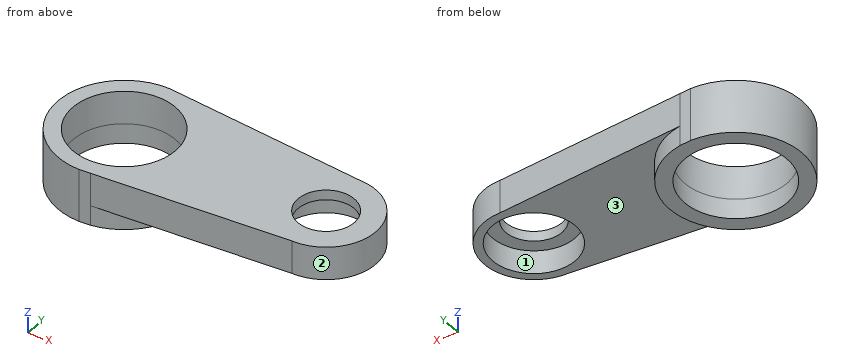
```python
from build123d import *

# Parameters (mm, degrees)
F0_R     = 7.75
F0_R_2   = 6.25
F0_R_3   = 4.25
F1_DEPTH = 5
F2_DEPTH = 3
F3_DEPTH = 3.5


with BuildPart() as f1:
    # F0 (on Top) → F1 (new body)
    with BuildSketch(Plane.XY):
        with BuildLine():
            Line((1.6551724138, 9.8620689655), (0, 10))
            ThreePointArc((0, 10), (-10, 0), (0, -10))
            Line((0, -10), (1.6551724138, -9.8620689655))
            ThreePointArc((1.6551724138, -9.8620689655), (7.6338628537, -6.4594224147), (10, 0))
            ThreePointArc((10, 0), (7.6338628537, 6.4594224147), (1.6551724138, 9.8620689655))
        make_face()
        Circle(F0_R, mode=Mode.SUBTRACT)
        with BuildLine():
            Line((30, 7.5), (1.6551724138, 9.8620689655))
            ThreePointArc((1.6551724138, 9.8620689655), (7.6338628537, 6.4594224147), (10, 0))
            ThreePointArc((10, 0), (7.6338628537, -6.4594224147), (1.6551724138, -9.8620689655))
            Line((1.6551724138, -9.8620689655), (30, -7.5))
            ThreePointArc((30, -7.5), (22.5, 0), (30, 7.5))
        make_face()
        with BuildLine():
            ThreePointArc((37.5, 0), (35.3033008589, 5.3033008589), (30, 7.5))
            ThreePointArc((30, 7.5), (22.5, 0), (30, -7.5))
            ThreePointArc((30, -7.5), (35.3033008589, -5.3033008589), (37.5, 0))
        make_face()
        with Locations((30, 0)):
            Circle(F0_R_2, mode=Mode.SUBTRACT)
        with Locations((30, 0)):
            Circle(F0_R_2)
        with Locations((30, 0)):
            Circle(F0_R_3, mode=Mode.SUBTRACT)
    extrude(amount=F1_DEPTH)

    # F0 (on Top) → F2 (join)
    with BuildSketch(Plane.XY):
        with BuildLine():
            Line((1.6551724138, 9.8620689655), (0, 10))
            ThreePointArc((0, 10), (-10, 0), (0, -10))
            Line((0, -10), (1.6551724138, -9.8620689655))
            ThreePointArc((1.6551724138, -9.8620689655), (7.6338628537, -6.4594224147), (10, 0))
            ThreePointArc((10, 0), (7.6338628537, 6.4594224147), (1.6551724138, 9.8620689655))
        make_face()
        Circle(F0_R, mode=Mode.SUBTRACT)
    extrude(amount=-F2_DEPTH)

    # F0 (on Top) → F3 (cut)
    with BuildSketch(Plane.XY):
        with Locations((30, 0)):
            Circle(F0_R_2)
        with Locations((30, 0)):
            Circle(F0_R_3, mode=Mode.SUBTRACT)
    extrude(amount=F3_DEPTH, mode=Mode.SUBTRACT)


solid = f1.part
```
Read the model definition and answer for the solid it produces. Units are mm, in the model's axes. Face numbers are marked on the shaded views. Give positions to 0.01 mm unless a question says otherwise; leave off trailing zeros. Write each loop counter-clockwise with the first axis right and the second up, starting at its lowest first coordinate (ties: lowest second). Pieces come first, ordered by that corner, then holes. Notation, with made-up numbers: (62, 65.25) -> (115, 65.25) arc R17 ccw to (115, 90.25) -> close; hole circle Ø2 at (73.25, 18). An arc over 180 degrees is marked (long way). Answer in a Markdown table with one row per item.
1) Section D-D on z = -1.5 is taken. Give the vertices of the cut face in (x, y), plus the area to 3 significant figures.
Results list:
| item | result |
|---|---|
| outline | (0, -10) -> (1.66, -9.86) arc R10 ccw to (1.66, 9.86) -> (0, 10) arc R10 ccw to start; hole circle Ø15.5 at (0, 0) |
| area | 125 mm^2 |
2) Section A-A on z = 0.5 is taken. Give the vertices of the cut face in (x, y), plus the area to 3 significant figures.
Results list:
| item | result |
|---|---|
| outline | (0, -10) -> (30, -7.5) arc R7.5 ccw to (30, 7.5) -> (0, 10) arc R10 ccw to start; hole circle Ø15.5 at (0, 0); hole circle Ø12.5 at (30, 0) |
| area | 459 mm^2 |
3) Straight lines are drawn through the part: line 1 (Y direction, x = 30, z = 2.3); line 2 (X direction, y = 5.75, z = 2.5); line 3 (X direction, y = -1.5, z = 0.25). For each, find the intervals that lie inside material, in ascending order. Write a range as [from, to].
Results list:
| item | result |
|---|---|
| line 1 | [-7.5, -6.25], [6.25, 7.5] |
| line 2 | [-8.18, -5.2], [5.2, 27.55], [32.45, 34.82] |
| line 3 | [-9.89, -7.6], [7.6, 23.93], [36.07, 37.35] |
4) Section B-B on y = 2.25 is taken. Give the vertices of the cut face in (x, z).
Results list:
| item | result |
|---|---|
| outline | (-9.74, -3) -> (-7.42, -3) -> (-7.42, 5) -> (-9.74, 5) -> close; (7.42, -3) -> (9.74, -3) -> (9.74, 0) -> (24.17, 0) -> (24.17, 3.5) -> (26.39, 3.5) -> (26.39, 5) -> (7.42, 5) -> close; (33.61, 3.5) -> (35.83, 3.5) -> (35.83, 0) -> (37.15, 0) -> (37.15, 5) -> (33.61, 5) -> close |
5) Each of these flat-tipped pins is pushed along its axis until it touches: pin 1 Ø4 at (x, z) = (-3.5, -0.5) entering from -Y; pin 2 Ø4 at (x, y) = (18, -6.5) entering from -Z; pin 3 Ø1.5 at (y, z) = (5, 0) entering from +X. Where does it stop, or does it pass through?
Results list:
| item | result |
|---|---|
| pin 1 | y = -9.89 |
| pin 2 | z = 0 |
| pin 3 | x = 36.18 |
6) Determine the mould class of the marked faces 1, 2 and 3 for opening direction Y: released by +Y, released by -Y, zero draft, split by the parting line, or undercut.
Results list:
| item | result |
|---|---|
| face 1 | undercut |
| face 2 | split by the parting line |
| face 3 | zero draft |
7) Section C-C on x = -2 is taken. Give the vertices of the cut face in (y, z).
Results list:
| item | result |
|---|---|
| outline | (-9.8, -3) -> (-7.49, -3) -> (-7.49, 5) -> (-9.8, 5) -> close; (7.49, -3) -> (9.8, -3) -> (9.8, 5) -> (7.49, 5) -> close |
